```python
from build123d import *

# Parameters (mm, degrees)
ESQUISSE1_W             = 75
ESQUISSE1_H             = 75
ESQUISSE1_R             = 15
BOSS_EXTRU_2_DEPTH      = 10
ESQUISSE2_R             = 10.125
BOSS_EXTRU_3_DEPTH      = 75
ESQUISSE3_W             = 55
ESQUISSE3_H             = 122.401822982
ENL_V_MAT_EXTRU_1_DEPTH = 143.473736615
CONG_1_R                = 3


with BuildPart() as part:
    # Esquisse1 → Boss.-Extru.2 (new body)
    with BuildSketch(Plane(origin=(0, 0, 0), x_dir=(1, 0, 0), z_dir=(0, 1, 0))):
        with Locations((37.5, 37.5)):
            Rectangle(ESQUISSE1_W, ESQUISSE1_H)
        with Locations(Location((37.5, 37.5, 0), (0, 0, 270))):
            Circle(ESQUISSE1_R, mode=Mode.SUBTRACT)
    extrude(amount=BOSS_EXTRU_2_DEPTH)

    # Esquisse2 → Boss.-Extru.3 (add)
    with BuildSketch(Plane(origin=(75, 0, 0), x_dir=(0, 0, -1), z_dir=(1, 0, 0))):
        with BuildLine():
            Line((62.145999584, 74.88265599), (75, 10))
            Line((75, 10), (0, 10))
            Line((0, 10), (12.854000416, 74.88265599))
            ThreePointArc((12.854000416, 74.88265599), (37.5, 95.125), (62.145999584, 74.88265599))
        make_face()
        with Locations((37.5, 70)):
            Circle(ESQUISSE2_R, mode=Mode.SUBTRACT)
    extrude(amount=-BOSS_EXTRU_3_DEPTH)

    # Esquisse3 → Enlèv. mat.-Extru.1 (cut, through all)
    with BuildSketch(Plane.XY):
        with Locations((37.5, 71.200911491)):
            Rectangle(ESQUISSE3_W, ESQUISSE3_H)
    extrude(amount=-ENL_V_MAT_EXTRU_1_DEPTH, mode=Mode.SUBTRACT)

    # Congé1
    cong_1_edges = [part.edges().sort_by_distance(p)[0] for p in [
        (10, 10, -37.5),
        (65, 10, -37.5),
    ]]
    fillet(cong_1_edges, radius=CONG_1_R)


solid = part.part
```
Input: part model. Units: mm. Frame: model coordinates. A direction names the side the tool comes from. Give positions to 0.01 mm unless a question says otherwise; leave off trailing zeros. Loops run counter-clockwise (first coordinate to the right, second up) from the corner with the lowest first, then second, coordinate; pieces in that order, holes last.
1) Section query D-D on y = 51.5. Return the cut outline in (x, z).
A:
outline: (0, -66.78) - (10, -66.78) - (10, -8.22) - (0, -8.22) - close; (65, -66.78) - (75, -66.78) - (75, -8.22) - (65, -8.22) - close
2) Line query: L1, parallel to Y at x = 4.75, z = -37.5 (3 decimals); L2, parallel to Z at x = 37, y = 2; L3, parallel to X at y = 6, z = -37. Output: solid intervals per line, ascending.
A:
L1: y = 0 to 59.875, 80.125 to 95.125
L2: z = -75 to -52.49, -22.51 to 0
L3: x = 0 to 22.51, 52.49 to 75
3) Reachability of faces 4 (the cylindrical face through (64.14, 10.9, -38.03)), 5 (the flat face through (5.147, 42.896, -68.483)) from +Z, -Z, +X, -X, +Y, -Y: full face, straight path, thin tool, end or side. Return the list, or none.
A:
face 4: +Z, -Z, +Y
face 5: -Z, +X, -X, +Y
4) Section query A-A on x = 37.5. Return the cut outline in (y, z).
A:
outline: (0, -75) - (10, -75) - (10, -52.5) - (0, -52.5) - close; (0, -22.5) - (10, -22.5) - (10, 0) - (0, 0) - close
5) Contact query for flat-ended pins moving along their axis: pin 1 (1.5 mm diameter, centred on x = 51.5, z = -34, fed in from +Y); pin 2 (4 mm diameter, centred on x = 66, y = 54.5, fed in from -Z); pin 3 (6 mm diameter, centred on x = 12, y = 44.5, fed in from +Z). Output: stop coordinate, or through.
A:
pin 1: stops at y = 10
pin 2: stops at z = -66.58
pin 3: stops at z = -6.39
6) Mould query, pull axis Y, two halves, no side actions, for faces 1 (the cylindrical face through (10.9, 10.86, -38.02)), 2 (the flat face through (37, 5, -75)), 3 (the cylindrical face through (5.07, 70.445, -27.385)). Classes: released by +Y, released by -Y, zero draft, split by the parting line, or undercut.
A:
face 1: released by +Y
face 2: zero draft
face 3: undercut
7) Section query C-C on x = 68.5. Return the cut outline in (y, z) (3 decimals), and give its area (3 significant figures).
A:
outline: (0, -75) - (10, -75) - (74.883, -62.146) arc R25.125 ccw to (74.883, -12.854) - (10, 0) - (0, 0) - close; hole circle Ø20.25 at (70, -37.5)
area: 5,210 mm2
8) Section query B-B on z = -37.5. Return the cut outline in (x, y) (3 decimals).
A:
outline: (0, 0) - (22.5, 0) - (22.5, 10) - (13, 10) arc R3 cw to (10, 13) - (10, 59.875) - (0, 59.875) - close; (0, 80.125) - (10, 80.125) - (10, 95.125) - (0, 95.125) - close; (52.5, 0) - (75, 0) - (75, 59.875) - (65, 59.875) - (65, 13) arc R3 cw to (62, 10) - (52.5, 10) - close; (65, 80.125) - (75, 80.125) - (75, 95.125) - (65, 95.125) - close
